Autodesk Inventor part; units mm, degrees
ref_plane "4dummy_XY" through (0, 0, 0) normal (1, 0, 0) x (0, 0, -1)
ref_plane "4dummy_YZ" through (0, 0, 0) normal (0, 0, -1) x (0, 1, 0)
ref_plane "4dummy_ZX" through (0, 0, 0) normal (0, 1, 0) x (1, 0, 0)
sketch "Sketch_18" plane through (-20, 0, 0) normal (1, 0, 0) x (0, 0, -1)
  line L0 (-17, 1.5) -> (-15.5, 0)
  line L1 (-15.5, 0) -> (-8.745, 0)
  line L2 (-8.745, 0) -> (-8.245, 0.5)
  line L3 (-8.245, 0.5) -> (-3.75, 0.5)
  line L4 (-3.75, 0.5) -> (-3.25, 0)
  line L5 (-3.25, 0) -> (3.25, 0)
  line L6 (3.25, 0) -> (3.75, 0.5)
  line L7 (3.75, 0.5) -> (8.245, 0.5)
  line L8 (8.245, 0.5) -> (8.745, 0)
  line L9 (8.745, 0) -> (15.5, 0)
  line L10 (15.5, 0) -> (17, 1.5)
  line L11 (17, 1.5) -> (17, 7.0002)
  line L12 (17, 7.0002) -> (11.8003, 12.1999)
  line L13 (11.8003, 12.1999) -> (11.8003, 17.6796)
  line L14 (11.8003, 17.6796) -> (13.6381, 19.5174)
  arc A0 (16.4816, 22.3609) -> (13.6381, 19.5174) centre (16.9102, 19.0889) ccw
  line L15 (16.4816, 22.3609) -> (17, 22.8793)
  line L16 (17, 22.8793) -> (17, 25.1102)
  line L17 (17, 25.1102) -> (16.4686, 25.6415)
  arc A1 (13.6398, 28.4703) -> (16.4686, 25.6415) centre (16.9102, 28.9119) ccw
  line L18 (13.6398, 28.4703) -> (13.1102, 29)
  line L19 (13.1102, 29) -> (-13.1102, 29)
  line L20 (-13.1102, 29) -> (-13.6398, 28.4703)
  arc A2 (-16.4686, 25.6415) -> (-13.6398, 28.4703) centre (-16.9102, 28.9119) ccw
  line L21 (-16.4686, 25.6415) -> (-17, 25.1102)
  line L22 (-17, 25.1102) -> (-17, 22.8793)
  line L23 (-17, 22.8793) -> (-16.4816, 22.3609)
  arc A3 (-13.6381, 19.5174) -> (-16.4816, 22.3609) centre (-16.9102, 19.0889) ccw
  line L24 (-13.6381, 19.5174) -> (-11.8003, 17.6796)
  line L25 (-11.8003, 17.6796) -> (-11.8003, 12.1999)
  line L26 (-11.8003, 12.1999) -> (-17, 7.0002)
  line L27 (-17, 7.0002) -> (-17, 1.5)
extrude "Extrusion1" add sketch "Sketch_18" along normal mid plane 914.4
sketch "Sketch2" plane through (-477.2, 29, 13.1102) normal (0, 1, 0) x (1, 0, 0)
  point P0 (20, 13.1102)
hole "Hole1" at (-457.2, 29, 0) direction (0, -1, 0) diameter 9 depth 29 counterbore diameter 14 counterbore depth 12
pattern_linear "Rectangular Pattern1" count 4 spacing 80 along (1, 0, 0) of "Hole1"
ref_plane "4dummy_XY" through (0, 0, 0) normal (1, 0, 0) x (0, 0, -1)
ref_plane "4dummy_YZ" through (0, 0, 0) normal (0, 0, -1) x (0, 1, 0)
ref_plane "4dummy_ZX" through (0, 0, 0) normal (0, 1, 0) x (1, 0, 0)
ref_plane "4slide_XY" through (-20, 7.5, 0) normal (1, 0, 0) x (0, 0, -1)
ref_plane "4slide_YZ" through (-20, 7.5, 0) normal (0, 0, -1) x (0, 1, 0)
ref_plane "4slide_ZX" through (-20, 7.5, 0) normal (0, 1, 0) x (1, 0, 0)
ref_plane "4track_XY" through (0, 0, 0) normal (0, 0, 1) x (1, 0, 0)
ref_plane "4track_YZ" through (0, 0, 0) normal (1, 0, 0) x (0, 1, 0)
ref_plane "4track_ZX" through (0, 0, 0) normal (0, 1, 0) x (0, 0, 1)
properties part number "HSR35R128020 Rail"
Verification items for the finished model (mm, model axes). A direction names the side the tool comes from. Give positions to 0.01 mm unless a question says otherwise; leave off trailing zeros. Answer in a Markdown table with one row per item. Add a question column.
Item 1: Mould release check, pull along Z, two halves, no side actions. Record for faces 1 (the flat face through (-377, 17, 5)), 2 (the flat face through (-26, 29, 0)): released by +Z, released by -Z, zero draft, split by the parting line, or undercut.
Item 2: Gauge pin test, flat ends, axial feed: pin 1 (1.3 mm diameter, centred on x = -99.5, z = 7, fed in from -Y); pin 2 (6 mm diameter, centred on x = -17.5, y = 15, fed in from +Z); pin 3 (11.5 mm diameter, centred on x = -297.2, z = 0, fed in from +Y). Record the tip position at first contact, or that the pin passes through.
Item 3: Tool access check on faces 3 (the flat face through (-477.2, 15, 0)), 4 (the cylindrical face through (-450.366, 22.916, -1.517)). Record the directions out of +Z, -Z, +X, -X, +Y, -Y that give a thin tool (end or side, any length) a straight path to the whole face; none if there is none.
Item 4: Scan lines: probe 1 along X at (y, z) = (8.5, 0); probe 2 along X at (y, z) = (24, 0); probe 3 along Z at (x, y) = (-377.2, 10.5). Record each from-to range of solid material in increasing order. Write a range as from..to.
Filled sheet:
| question | item | result |
|---|---|---|
| 1 | face 1 | undercut |
| 1 | face 2 | zero draft |
| 2 | pin 1 | stops at y = 0.5 |
| 2 | pin 2 | stops at z = 12.12 |
| 2 | pin 3 | stops at y = 17 |
| 3 | face 3 | +Z, -Z, -X, +Y, -Y |
| 3 | face 4 | +Y |
| 4 | probe 1 | x = -477.2..-461.7, -452.7..-381.7, -372.7..-301.7, -292.7..-221.7, -212.7..437.2 |
| 4 | probe 2 | x = -477.2..-464.2, -450.2..-384.2, -370.2..-304.2, -290.2..-224.2, -210.2..437.2 |
| 4 | probe 3 | z = -13.5..-4.5, 4.5..13.5 |
